Geometry check sheet. Reference: the model listing, model coordinates, mm. Give positions to 0.01 mm unless a question says otherwise; leave off trailing zeros. Write each loop counter-clockwise with the first axis right and the second up, starting at its lowest first coordinate (ties: lowest second). Pieces come first, ordered by that corner, then holes. Notation, with made-up numbers: (13, 0.5) -> (53, 0.5) arc R6 ccw to (53, 8.5) -> close; hole circle Ø6 at (-16, -18). An arc over 180 degrees is marked (long way). One line per item, written item: value.
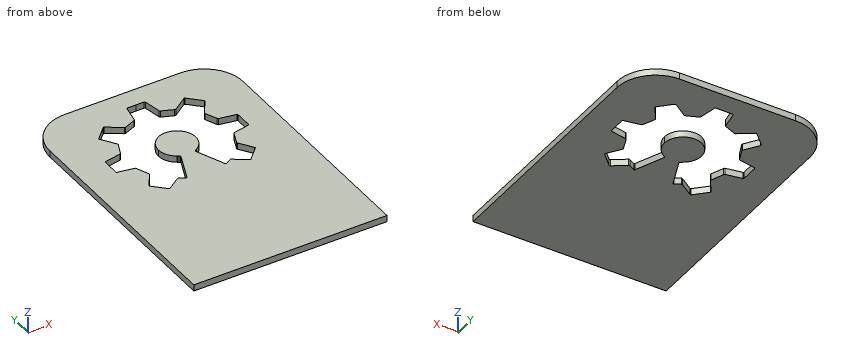
Autodesk Inventor part; units mm, degrees
ref_plane "YZ Plane" through (0, 0, 0) normal (1, 0, 0) x (0, 1, 0)
ref_plane "XZ Plane" through (0, 0, 0) normal (0, 1, 0) x (-1, 0, 0)
ref_plane "XY Plane" through (0, 0, 0) normal (0, 0, 1) x (1, 0, 0)
sketch "Sketch1" plane through (0, 0, 0) normal (0, 0, 1) x (1, 0, 0)
  line L0 (-15, -18) -> (15, -18)
  line L1 (15, -18) -> (15, 18)
  line L2 (9, 24) -> (-9, 24)
  line L3 (-15, 18) -> (-15, -18)
  arc A0 (-9, 24) -> (-15, 18) centre (-9, 18) ccw
  arc A1 (15, 18) -> (9, 24) centre (9, 18) ccw
  point P0 (0, 0)
  point P1 (15, 24)
  point P2 (-15, 24)
  point P3 (15, 0)
  point P4 (0, 24)
  dimension "d0" = 30
  dimension "d1" = 42
  dimension "d2" = 6
extrude "Extrusion1" add sketch "Sketch1" along normal blind 1
sketch "Sketch2" plane through (0, 0, 0) normal (0, 0, 1) x (1, 0, 0)
  arc A0 (-3.8619, 17.3067) -> (-3.6654, 17.2925) centre (-3.7499, 17.4911) ccw
  line L0 (-3.6654, 17.2925) -> (-1.9114, 18.0105)
  arc A1 (-1.9114, 18.0105) -> (-1.782, 18.1586) centre (-1.9892, 18.209) ccw
  line L1 (-1.782, 18.1586) -> (-1.2951, 20.7754)
  arc A2 (-1.1603, 20.8876) -> (-1.2951, 20.7754) centre (-1.1555, 20.7447) ccw
  line L2 (-1.1603, 20.8876) -> (0.1418, 20.8876)
  arc A3 (3.0232, 10.5703) -> (-2.7384, 10.57) centre (0.1424, 10.5701) ccw
  arc A4 (-2.7384, 10.57) -> (-1.4094, 8.1444) centre (0.1397, 10.5701) ccw
  arc A5 (-1.4094, 8.1444) -> (-1.2693, 8.0371) centre (-0.717, 8.9031) ccw
  line L3 (-1.2693, 8.0371) -> (-1.0511, 7.9035)
  line L4 (-0.9944, 7.7366) -> (-2.8191, 3.3275)
  arc A6 (-2.9648, 3.2741) -> (-2.8191, 3.3275) centre (-2.9158, 3.3658) ccw
  line L5 (-2.9648, 3.2741) -> (-3.8472, 3.7453)
  arc A7 (-3.8472, 3.7453) -> (-4.0418, 3.7399) centre (-3.9398, 3.572) ccw
  line L6 (-4.0418, 3.7399) -> (-6.0484, 2.3626)
  arc A8 (-6.2232, 2.3788) -> (-6.0484, 2.3626) centre (-6.1253, 2.4841) ccw
  line L7 (-6.2232, 2.3788) -> (-8.061, 4.2166)
  arc A9 (-8.0807, 4.3951) -> (-8.061, 4.2166) centre (-7.9596, 4.3181) ccw
  line L8 (-8.0807, 4.3951) -> (-6.6787, 6.4378)
  arc A10 (-6.6787, 6.4378) -> (-6.6624, 6.6306) centre (-6.8628, 6.5504) ccw
  line L9 (-6.6624, 6.6306) -> (-7.436, 8.5631)
  arc A11 (-7.436, 8.5631) -> (-7.581, 8.6886) centre (-7.6302, 8.4854) ccw
  line L10 (-7.581, 8.6886) -> (-10.0488, 9.1479)
  arc A12 (-10.161, 9.2831) -> (-10.0488, 9.1479) centre (-10.0181, 9.2876) ccw
  line L11 (-10.161, 9.2831) -> (-10.1612, 11.8869)
  arc A13 (-10.049, 12.0221) -> (-10.1612, 11.8869) centre (-10.018, 11.8822) ccw
  line L12 (-10.049, 12.0221) -> (-7.5191, 12.4926)
  arc A14 (-7.5191, 12.4926) -> (-7.3693, 12.6214) centre (-7.5703, 12.7036) ccw
  line L13 (-7.3693, 12.6214) -> (-6.5937, 14.4306)
  arc A15 (-6.5937, 14.4306) -> (-6.6058, 14.6262) centre (-6.7865, 14.5168) ccw
  line L14 (-6.6058, 14.6262) -> (-8.0801, 16.7747)
  arc A16 (-8.0639, 16.9496) -> (-8.0801, 16.7747) centre (-7.9592, 16.8517) ccw
  line L15 (-8.0639, 16.9496) -> (-6.2228, 18.7908)
  arc A17 (-6.048, 18.8069) -> (-6.2228, 18.7908) centre (-6.125, 18.6867) ccw
  line L16 (-6.048, 18.8069) -> (-3.8619, 17.3067)
  arc A18 (-0.9944, 7.7366) -> (-1.0511, 7.9035) centre (-1.1231, 7.786) ccw
  line L17 (0.1418, 20.8876) -> (0.1429, 2.0479) construction
  arc A19 (2.0659, 18.1588) -> (2.1953, 18.0107) centre (2.2731, 18.2093) ccw
  line L18 (2.0659, 18.1588) -> (1.5788, 20.7755)
  arc A20 (1.6945, 8.1446) -> (3.0232, 10.5703) centre (0.145, 10.5701) ccw
  arc A21 (1.5544, 8.0373) -> (1.6945, 8.1446) centre (1.002, 8.9032) ccw
  line L19 (1.5544, 8.0373) -> (1.3362, 7.9037)
  line L20 (1.2795, 7.7367) -> (3.1047, 3.3278)
  line L21 (8.3662, 4.3961) -> (6.964, 6.4386)
  arc A22 (8.3466, 4.2175) -> (8.3662, 4.3961) centre (8.2451, 4.319) ccw
  arc A23 (4.3274, 3.7404) -> (4.1328, 3.7458) centre (4.2254, 3.5724) ccw
  line L22 (3.2504, 3.2745) -> (4.1328, 3.7458)
  arc A24 (3.1047, 3.3278) -> (3.2504, 3.2745) centre (3.2014, 3.3662) ccw
  line L23 (4.3274, 3.7404) -> (6.3342, 2.3633)
  arc A25 (6.3342, 2.3633) -> (6.509, 2.3795) centre (6.411, 2.4848) ccw
  line L24 (6.509, 2.3795) -> (8.3466, 4.2175)
  line L25 (10.3336, 12.0232) -> (7.8037, 12.4935)
  arc A26 (10.4458, 11.8881) -> (10.3336, 12.0232) centre (10.3027, 11.8834) ccw
  arc A27 (7.866, 8.6895) -> (7.7211, 8.564) centre (7.9152, 8.4863) ccw
  arc A28 (10.3338, 9.1491) -> (10.446, 9.2843) centre (10.3031, 9.2887) ccw
  line L26 (7.866, 8.6895) -> (10.3338, 9.1491)
  line L27 (6.9477, 6.6314) -> (7.7211, 8.564)
  arc A29 (6.9477, 6.6314) -> (6.964, 6.4386) centre (7.148, 6.5512) ccw
  line L28 (10.446, 9.2843) -> (10.4458, 11.8881)
  arc A30 (3.9494, 17.293) -> (4.1459, 17.3071) centre (4.0339, 17.4915) ccw
  line L29 (3.9494, 17.293) -> (2.1953, 18.0107)
  arc A31 (7.6539, 12.6222) -> (7.8037, 12.4935) centre (7.8549, 12.7045) ccw
  line L30 (7.6539, 12.6222) -> (6.878, 14.4314)
  arc A32 (6.8902, 14.627) -> (6.878, 14.4314) centre (7.0708, 14.5176) ccw
  line L31 (6.8902, 14.627) -> (8.3642, 16.7757)
  arc A33 (8.3642, 16.7757) -> (8.348, 16.9506) centre (8.2433, 16.8527) ccw
  line L32 (1.4439, 20.8877) -> (0.1418, 20.8876)
  arc A34 (1.5788, 20.7755) -> (1.4439, 20.8877) centre (1.4392, 20.7449) ccw
  line L33 (6.3318, 18.8076) -> (4.1459, 17.3071)
  arc A35 (1.3362, 7.9037) -> (1.2795, 7.7367) centre (1.4082, 7.7861) ccw
  line L34 (8.348, 16.9506) -> (6.5066, 18.7915)
  arc A36 (6.5066, 18.7915) -> (6.3318, 18.8076) centre (6.4089, 18.6874) ccw
  point P0 (0, 0)
  point P1 (0.145, 10.5701)
  point P2 (0.145, 10.5701)
  point P3 (0.145, 10.5701)
  dimension "d5" = 18.525
extrude "Extrusion2" cut sketch "Sketch2" along normal blind 1
properties part number "VerticalPiece"
1) Sectioned sample at C-C on x = 5.75. Record the cut outline in (y, z), plus the area to 3 significant figures.
Verdict:
outline: (-18, 0) -> (2.76, 0) -> (2.76, 1) -> (-18, 1) -> close; (18.41, 0) -> (24, 0) -> (24, 1) -> (18.41, 1) -> close
area: 26.4 mm^2
2) Sectioned sample at B-B on y = 5. Record the cut outline in (x, z), plus the area to 3 significant figures.
Verdict:
outline: (-15, 0) -> (-7.67, 0) -> (-7.67, 1) -> (-15, 1) -> close; (-2.13, 0) -> (2.41, 0) -> (2.41, 1) -> (-2.13, 1) -> close; (7.95, 0) -> (15, 0) -> (15, 1) -> (7.95, 1) -> close
area: 18.9 mm^2
3) Sectioned sample at A-A on x = -0.5. Record the cut outline in (y, z).
Verdict:
outline: (-18, 0) -> (13.38, 0) -> (13.38, 1) -> (-18, 1) -> close; (20.89, 0) -> (24, 0) -> (24, 1) -> (20.89, 1) -> close
4) Scan lines: probe 1 along X at (y, z) = (10.5, 0.1); probe 2 along Y at (x, z) = (7.5, 0.1); probe 3 along X at (y, z) = (18, 0.65). Record each from-to range of solid material in increasing order.
Verdict:
probe 1: -15 to -10.16, -2.74 to 3.02, 10.45 to 15
probe 2: -18 to 3.37, 5.66 to 8.01, 12.98 to 15.52, 17.8 to 24
probe 3: -15 to -7.01, -4.87 to -1.94, 2.22 to 5.16, 7.3 to 15
5) Sectioned sample at D-D on x = -12. Record the cut outline in (y, z), plus the area to 3 significant figures.
Verdict:
outline: (-18, 0) -> (23.2, 0) -> (23.2, 1) -> (-18, 1) -> close
area: 41.2 mm^2
